Geometry: final body of the model. Coordinates: model frame, mm. A direction names the side the tool comes from. Coordinates: 2 decimals unless noted, no trailing zeros. Write each loop counter-clockwise with the first axis right and the second up, starting at its lowest first coordinate (ties: lowest second). Pieces come first, ordered by that corner, then holes. Notation, with made-up numbers: (67.25, 51) - (100.25, 51) arc R23 ccw to (100.25, 80) - close; hole circle Ø4 at (81.5, 88.25). An arc over 180 degrees is marked (long way). Answer as a JSON object with one key per item and string values. Group by question number.
Item 1: Section D-D on x = -4.25. Return loops of the section in (y, z), and give its area (3 significant figures).
Item 2: Section A-A on z = 2. Return loops of the section in (x, y), and give its area (3 significant figures).
Item 3: Set-up query: faces 1 (the flat face through (-4, 5, 0)), 2 (the cylindrical face through (-5.289, -5.986, 4.196)). Return all of +Z, -Z, +X, -X, +Y, -Y with unobstructed straight access to the full face (end or side cutting, diameter ignored); none if empty.
Item 4: Mould query, pull axis Z, two halves, no side actions, for faces 3 (the cylindrical face through (2.5, 5.9, -0.1)), 4 (the flat face through (5.1, 1.1, -6)), 5 (the flat face through (-4, 7, 0)), 6 (the cylindrical face through (2.5, -5.9, 0.1)). Classes: pulls with the +Z half, pulls with the -Z half, needs draft (parallel to the pull), parting line crosses it, or undercut.
Item 5: Section B-B on x = -0.5. Return loops of the section in (y, z), and give its area (3 significant figures).
Item 6: First-contact query: pin 1 Ø5 at (x, z) = (3, 0.5) entering from -Y; pin 2 Ø1 at (x, z) = (1.5, -3.5) entering from +Y; pin 3 Ø1 at (x, z) = (4, -4.5) entering from -Y. Flat tips, straight axial feed; report the tip coordinate or a pass-through.
Item 7: Line query: line 1 along Y through (x, z) = (-3.5, -2); line 2 along X through (y, z) = (-5.5, 0); line 3 along Z through (x, y) = (0, -5.5). Output: solid intervals per line, ascending. Write a range as from..to.
Autodesk Inventor part; units mm, degrees
ref_plane "YZ Plane" through (0, 0, 0) normal (1, 0, 0) x (0, 1, 0)
ref_plane "XZ Plane" through (0, 0, 0) normal (0, 1, 0) x (-1, 0, 0)
ref_plane "XY Plane" through (0, 0, 0) normal (0, 0, 1) x (1, 0, 0)
sketch "Sketch4" plane through (0, 0, 0) normal (0, 0, 1) x (1, 0, 0)
  arc A0 (0, -5) -> (0, 5) centre (0, 0) ccw
  line L0 (0, -5) -> (-7, -5)
  line L1 (-5, -5) -> (-5, 5) construction
  line L2 (-7, 5) -> (0, 5)
  line L3 (0, 5) -> (0, -5) construction
  arc A1 (-5, 0) -> (0, -5) centre (0, 0) ccw construction
  arc A2 (0, 5) -> (-5, 0) centre (0, 0) ccw construction
  arc A3 (-5, -4.899) -> (-4.899, -5) centre (0, 0) ccw construction
  line L4 (0, -7) -> (-7, -7)
  line L5 (-7, -7) -> (-7, -5)
  line L6 (-7, 7) -> (0, 7)
  arc A4 (-7, 0) -> (-5, -4.899) centre (0, 0) ccw construction
  arc A5 (-5, 4.899) -> (-7, 0) centre (0, 0) ccw construction
  arc A6 (-4.899, 5) -> (-5, 4.899) centre (0, 0) ccw construction
  arc A7 (0, 7) -> (-4.899, 5) centre (0, 0) ccw construction
  arc A8 (-4.899, -5) -> (0, -7) centre (0, 0) ccw construction
  arc A9 (0, -7) -> (0, 7) centre (0, 0) ccw
  line L7 (-7, -5) -> (-7, 5) construction
  line L8 (-7, 5) -> (-7, 7)
  dimension "d14" = 10
  dimension "d15" = 2
extrude "Extrusion4" add sketch "Sketch4" along normal mid plane 12
sketch "Sketch5" plane through (0, 0, 0) normal (0, 1, 0) x (-1, 0, 0)
  circle A0 centre (0, 0) radius 2.5
  dimension "d18" = 5
extrude "Extrusion5" cut sketch "Sketch5" along normal through all both and the other way through all
fillet "Fillet1" radius 6 4 edges at (-7, 6, 6) (-7, 6, -6) (-7, -6, -6) (-7, -6, 6)
properties part number "tip-protector" material "Rubber"
Checks:
{
 "1": {"outline": "(-7, -5.04) - (-5, -5.04) - (-5, 5.04) - (-7, 5.04) - close; (5, -5.04) - (7, -5.04) - (7, 5.04) - (5, 5.04) - close", "area": "40.4 mm^2"},
 "2": {"outline": "(-6.66, -7) - (-1.5, -7) - (-1.5, -5) - (-6.66, -5) - close; (-6.66, 5) - (-1.5, 5) - (-1.5, 7) - (-6.66, 7) - close; (1.5, -6.84) arc R7 ccw to (1.5, 6.84) - (1.5, 4.77) arc R5 cw to (1.5, -4.77) - close", "area": "52.3 mm^2"},
 "3": {"face 1": "+Z, -Z, -X", "face 2": "+Z, -X, +Y, -Y"},
 "4": {"face 3": "undercut", "face 4": "pulls with the -Z half", "face 5": "needs draft", "face 6": "undercut"},
 "5": {"outline": "(-7, -6) - (-5, -6) - (-5, -2.45) - (-7, -2.45) - close; (-7, 2.45) - (-5, 2.45) - (-5, 6) - (-7, 6) - close; (5, -6) - (7, -6) - (7, -2.45) - (5, -2.45) - close; (5, 2.45) - (7, 2.45) - (7, 6) - (5, 6) - close", "area": "28.4 mm^2"},
 "6": {"pin 1": "y = -6.9", "pin 2": "y = 6.93", "pin 3": "y = -6.06"},
 "7": {"line 1": "-7..-5, 5..7", "line 2": "-7..-2.5, 2.5..4.33", "line 3": "-6..-2.5, 2.5..6"}
}
